The listing builds one solid part. Answer for the finished solid, in the listing's coordinates (mm). A direction names the side the tool comes from. Coordinates: 2 decimals unless noted, no trailing zeros. Order: outer loops, then holes, each group sorted by start corner. A loop starts at its lowest first (then second) coordinate and runs counter-clockwise, first axis right, second up. Notation, with made-up numbers: M -39,13.25 L 15,13.25 A28 ccw 15,37.25 Z; hole C 39,54 d8. An arc over 180 degrees is marked long. One line per item, written item: value. Start each with the question number.
Q1. The part is cut by section B-B on x = 36. Give the vertices of the cut face in (y, z) (3 decimals), then the cut area to 3 significant figures.
Q2. Determine the mould class of faces 1 (the flat face through (23.175, 2, -3)), 2 (the flat face through (0, 2, -70)) for opening direction Z: pulls with the +Z half, pulls with the -Z half, needs draft (parallel to the pull), parting line crosses it, or undercut.
Q3. The part is cut by section D-D on x = 95.85. Give the number of separate pieces and of enclosed holes in the cut face, then the cut area to 3 significant figures.
Q4. The part is cut by section C-C on z = -10. Give the vertices of the cut face in (x, y) (3 decimals).
Q5. The part is cut by section A-A on z = -35. Give the vertices of the cut face in (x, y) (3 decimals), then the cut area to 3 significant figures.
Q6. Straight lines are drawn through the part: line 1 along X through (y, z) = (0.8, -10) (3 decimals); line 2 along X through (y, z) = (2.75, -56.5) (3 decimals); line 3 along Z through (x, y) = (64.5, 2.7). For each, find the intervals that lie inside material, in ascending order. Write a range as [from, to].
Q7. For faces 3 (the flat face through (88.35, 2, -150)), 4 (the flat face through (0, 2, -30)), 5 (the flat face through (0, 2, 3)), 6 (the flat face through (96, 2, -80)), 7 (the flat face through (21.147, 1.565, -79.823)), determine the directions among +Z, -Z, +X, -X, +Y, -Y from which every point of the face is accessible in a straight line to the end or side of a thin tool.
Q8. Each of these flat-tipped pins is pushed along its axis until it touches: pin 1 Ø1.6 at (x, y) = (-5, 1.5) entering from +Z; pin 2 Ø1.6 at (x, y) = (-9, 2) entering from -Z; pin 3 Ø1 at (x, y) = (41.5, 1) entering from +Z. Where does it stop, or does it pass through?
```python
from build123d import *

# Parameters (mm, degrees)
BOSS_EXTRUDE1_DEPTH = 3.175
SKETCH3_W           = 15
SKETCH3_H           = 20
SKETCH3_R           = 3.5
BOSS_EXTRUDE3_DEPTH = 3.175
SKETCH4_W           = 23.175
SKETCH4_H           = 6.096
BOSS_EXTRUDE4_DEPTH = 3.175


with BuildPart() as part:
    # Sketch1 → Boss-Extrude1 (new body)
    with BuildSketch(Plane(origin=(0, 0, 0), x_dir=(1, 0, 0), z_dir=(0, 1, 0))):
        Polygon((0, 160), (0, 0), (23.175, 0), (23.175, 12.666666667), (19.175, 25.333333333), (19.175, 67.333333333), (23.175, 92.666666667), (23.175, 134.666666667), (65.175, 134.666666667), (65.175, 92.666666667), (65.175, 88.666666667), (26.543421053, 88.666666667), (23.175, 67.333333333), (65.175, 67.333333333), (65.175, 25.333333333), (65.175, 0), (88.35, 0), (88.35, 160), align=None)
    extrude(amount=BOSS_EXTRUDE1_DEPTH)

    # Sketch3 → Boss-Extrude3 (add)
    # profile 1 of 8: a face of its own
    with BuildSketch(Plane(origin=(0, 3.175, 0), x_dir=(1, 0, 0), z_dir=(0, 1, 0))):
        with Locations((-7.5, 130)):
            Rectangle(SKETCH3_W, SKETCH3_H)
        with Locations(Location((-7.5, 130, 0), (0, 0, 270))):
            Circle(SKETCH3_R, mode=Mode.SUBTRACT)
    # profile 2 of 8: a face of its own
    with BuildSketch(Plane(origin=(0, 3.175, 0), x_dir=(1, 0, 0), z_dir=(0, 1, 0))):
        with Locations((-7.5, 90)):
            Rectangle(SKETCH3_W, SKETCH3_H)
        with Locations(Location((-7.5, 90, 0), (0, 0, 270))):
            Circle(SKETCH3_R, mode=Mode.SUBTRACT)
    # profile 3 of 8: a face of its own
    with BuildSketch(Plane(origin=(0, 3.175, 0), x_dir=(1, 0, 0), z_dir=(0, 1, 0))):
        with Locations((-7.5, 50)):
            Rectangle(SKETCH3_W, SKETCH3_H)
        with Locations(Location((-7.5, 50, 0), (0, 0, 270))):
            Circle(SKETCH3_R, mode=Mode.SUBTRACT)
    # profile 4 of 8: a face of its own
    with BuildSketch(Plane(origin=(0, 3.175, 0), x_dir=(1, 0, 0), z_dir=(0, 1, 0))):
        with Locations((-7.5, 10)):
            Rectangle(SKETCH3_W, SKETCH3_H)
        with Locations(Location((-7.5, 10, 0), (0, 0, 270))):
            Circle(SKETCH3_R, mode=Mode.SUBTRACT)
    # profile 5 of 8: a face of its own
    with BuildSketch(Plane(origin=(0, 3.175, 0), x_dir=(1, 0, 0), z_dir=(0, 1, 0))):
        with Locations((95.85, 10)):
            Rectangle(SKETCH3_W, SKETCH3_H)
        with Locations(Location((95.85, 10, 0), (0, 0, 270))):
            Circle(SKETCH3_R, mode=Mode.SUBTRACT)
    # profile 6 of 8: a face of its own
    with BuildSketch(Plane(origin=(0, 3.175, 0), x_dir=(1, 0, 0), z_dir=(0, 1, 0))):
        with Locations((95.85, 50)):
            Rectangle(SKETCH3_W, SKETCH3_H)
        with Locations(Location((95.85, 50, 0), (0, 0, 270))):
            Circle(SKETCH3_R, mode=Mode.SUBTRACT)
    # profile 7 of 8: a face of its own
    with BuildSketch(Plane(origin=(0, 3.175, 0), x_dir=(1, 0, 0), z_dir=(0, 1, 0))):
        with Locations((95.85, 90)):
            Rectangle(SKETCH3_W, SKETCH3_H)
        with Locations(Location((95.85, 90, 0), (0, 0, 270))):
            Circle(SKETCH3_R, mode=Mode.SUBTRACT)
    # profile 8 of 8: a face of its own
    with BuildSketch(Plane(origin=(0, 3.175, 0), x_dir=(1, 0, 0), z_dir=(0, 1, 0))):
        with Locations((95.85, 130)):
            Rectangle(SKETCH3_W, SKETCH3_H)
        with Locations(Location((95.85, 130, 0), (0, 0, 270))):
            Circle(SKETCH3_R, mode=Mode.SUBTRACT)
    extrude(amount=-BOSS_EXTRUDE3_DEPTH)

    # Sketch4 → Boss-Extrude4 (add)
    with BuildSketch(Plane(origin=(0, 3.175, 0), x_dir=(1, 0, 0), z_dir=(0, 1, 0))):
        with Locations((11.5875, -3.048)):
            Rectangle(SKETCH4_W, SKETCH4_H)
        with Locations((76.7625, -3.048)):
            Rectangle(SKETCH4_W, SKETCH4_H)
    extrude(amount=-BOSS_EXTRUDE4_DEPTH)


solid = part.part
```
Output:
1. outline: M 0,-160 L 3.175,-160 L 3.175,-134.667 L 0,-134.667 Z; M 0,-88.667 L 3.175,-88.667 L 3.175,-67.333 L 0,-67.333 Z
1. area: 148 mm^2
2. face 1: needs draft
2. face 2: undercut
3. separate pieces: 8
3. enclosed holes: 0
3. area: 165 mm^2
4. outline: M -15,0 L -11,0 L -11,3.175 L -15,3.175 Z; M -4,0 L 23.175,0 L 23.175,3.175 L -4,3.175 Z; M 65.175,0 L 92.35,0 L 92.35,3.175 L 65.175,3.175 Z; M 99.35,0 L 103.35,0 L 103.35,3.175 L 99.35,3.175 Z
5. outline: M 0,0 L 19.175,0 L 19.175,3.175 L 0,3.175 Z; M 65.175,0 L 88.35,0 L 88.35,3.175 L 65.175,3.175 Z
5. area: 134 mm^2
6. line 1: x = [-15, -11], [-4, 23.175], [65.175, 92.35], [99.35, 103.35]
6. line 2: x = [-15, 19.175], [65.175, 103.35]
6. line 3: z = [-160, -134.67], [-88.67, -67.33]
7. face 3: -Z, +X, +Y, -Y
7. face 4: -X, +Y, -Y
7. face 5: +Z, -X, +Y, -Y
7. face 6: +X, +Y, -Y
7. face 7: +Y, -Y
8. pin 1: stops at z = 0
8. pin 2: stops at z = -140
8. pin 3: stops at z = -67.33
